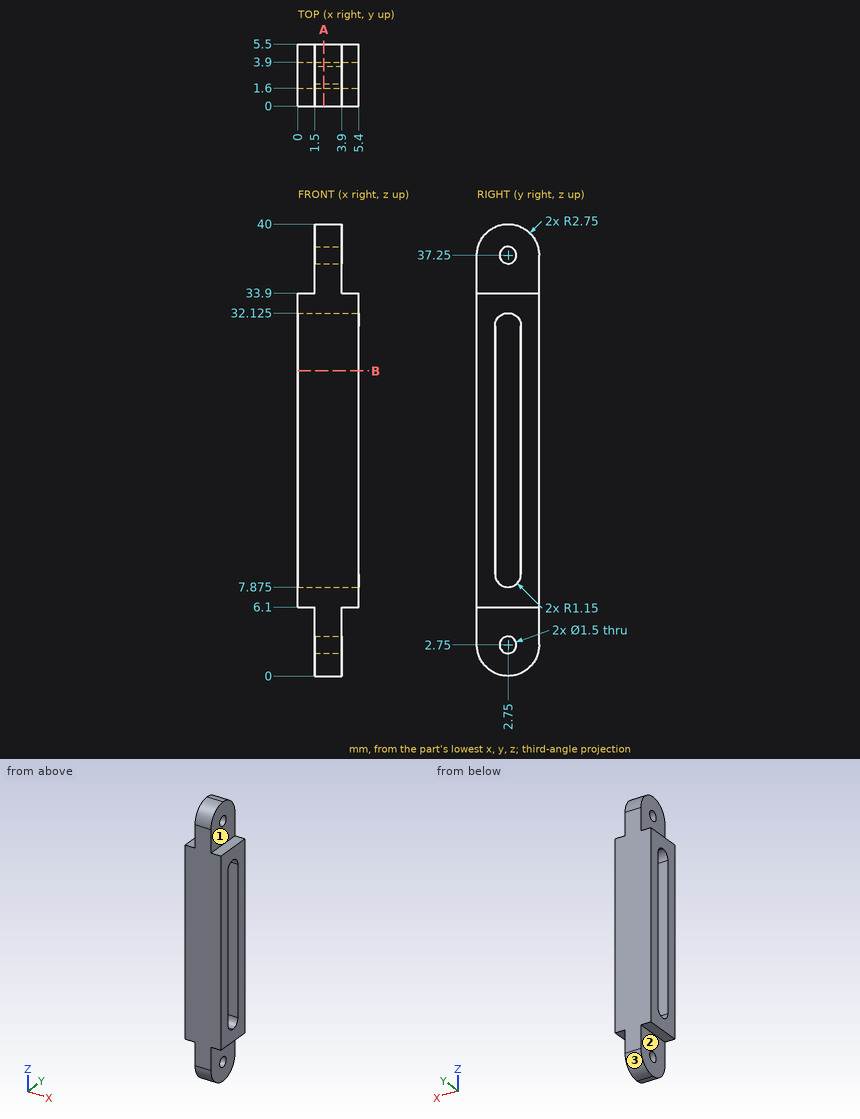
Geometry: see drawing. Coordinates: mm, zero at the bounding-box minimum. A direction names the side the tool comes from. Round coordinates to 2 decimals unless told otherwise and drop trailing zeros. Loops run counter-clockwise (first coordinate to the right, second up) from the corner with the lowest first, then second, coordinate; pieces in that order, holes last. Notation, with made-up numbers: (-6, 81.25) -> (2, 81.25) arc R14 cw to (2, 99.25) -> close; hole circle Ø9 at (-4, -2.5). An arc over 180 degrees is marked (long way). Use one line per item in the form item = value. Start each with the question number.
Item 1: Section query B-B on z = 27. Return the cut outline in (x, y).
Item 2: Set-up query: the marked faces 1, 2 and 3. Return all of +Z, -Z, +X, -X, +Y, -Y with unobstructed straight access to the full face (end or side cutting, diameter ignored); none if empty.
Item 3: Section query A-A on x = 2.3. Count the separate pieces of the cut face and the enclosed holes in it, then the cut area to 3 significant figures.
Item 4: Contact query for flat-ended pins moving along their axis: pin 1 Ø2 at (y, z) = (2.75, 37.25) entering from -X; pin 2 Ø1.5 at (y, z) = (2.5, 22.5) entering from +X; pin 3 Ø3 at (x, y) = (2.5, 4.5) entering from +Z; pin 4 Ø0.8 at (x, y) = (4.5, 3) entering from +Z. Output: stop coordinate, or through.
Item 5: Material intervals for L1, parallel to Y at x = 5.1, z = 27.5; L2, parallel to Z at x = 4.3, y = 2.75 (3 decimals); L3, parallel to X at y = 3.8, z = 34, sorted ascending. Write a range as from..to.
Ans:
q1.outline = (0, 0) -> (5.4, 0) -> (5.4, 1.6) -> (0, 1.6) -> close; (0, 3.9) -> (5.4, 3.9) -> (5.4, 5.5) -> (0, 5.5) -> close
q2.face_1 = +Z, +X, +Y, -Y
q2.face_2 = -Z, -X, +Y, -Y
q2.face_3 = -Z, +X, -X, +Y
q3.separate_pieces = 1
q3.enclosed_holes = 3
q3.area = 155 mm^2
q4.pin_1 = 1.5
q4.pin_2 = through
q4.pin_3 = 39.99
q4.pin_4 = 33.9
q5.L1 = 0..1.6, 3.9..5.5
q5.L2 = 6.1..7.875, 32.125..33.9
q5.L3 = 1.5..3.9
